Here's the drawing with two shaded views (mm, measured from the low corner). I have some questions. Coordinates: 2 decimals unless noted, no trailing zeros. Write each loop counter-clockwise with the first axis right and the second up, starting at its lowest first coordinate (ties: lowest second). Pieces come first, ordered by that corner, then holes. Notation, with made-up numbers: (72.25, -25.5) - (126.25, -25.5) arc R7 ccw to (126.25, -13.5) - close; hole circle Ø9 at (-4, 58). An arc over 180 degrees is marked (long way). Answer in a Markdown table with one row per item. Add a question column.
Item 1: If I drill on probe 1 along X at (y, z) = (1.9, 65); probe 2 along X at (y, z) = (2.1, 63); probe 3 along X at (y, z) = (1.65, 110), over which ranges is the centre line in solid material (lowest first)? Write a range as from..to.
Item 2: Imagine slicing it at A-A (x = 45). Please give me the cut outline in (y, z).
Item 3: Imagine slicing it at D-D (z = 14). Please give me the cut outline in (x, y), plus the area to 3 significant figures.
Item 4: Imagine slicing it at B-B (y = 2). State how many separate pieces and enclosed holes the cut face has, plus the area to 3 significant figures.
Item 5: I'm going to push a flat-ended pin straight in: pin 1 (10 mm diameter, centred on x = 34, z = 31.5, fed in from -Y). Where does the tip first touch, or does it pass through?
Item 6: Imagine slicing it at C-C (z = 65). Please give me the cut outline in (x, y).
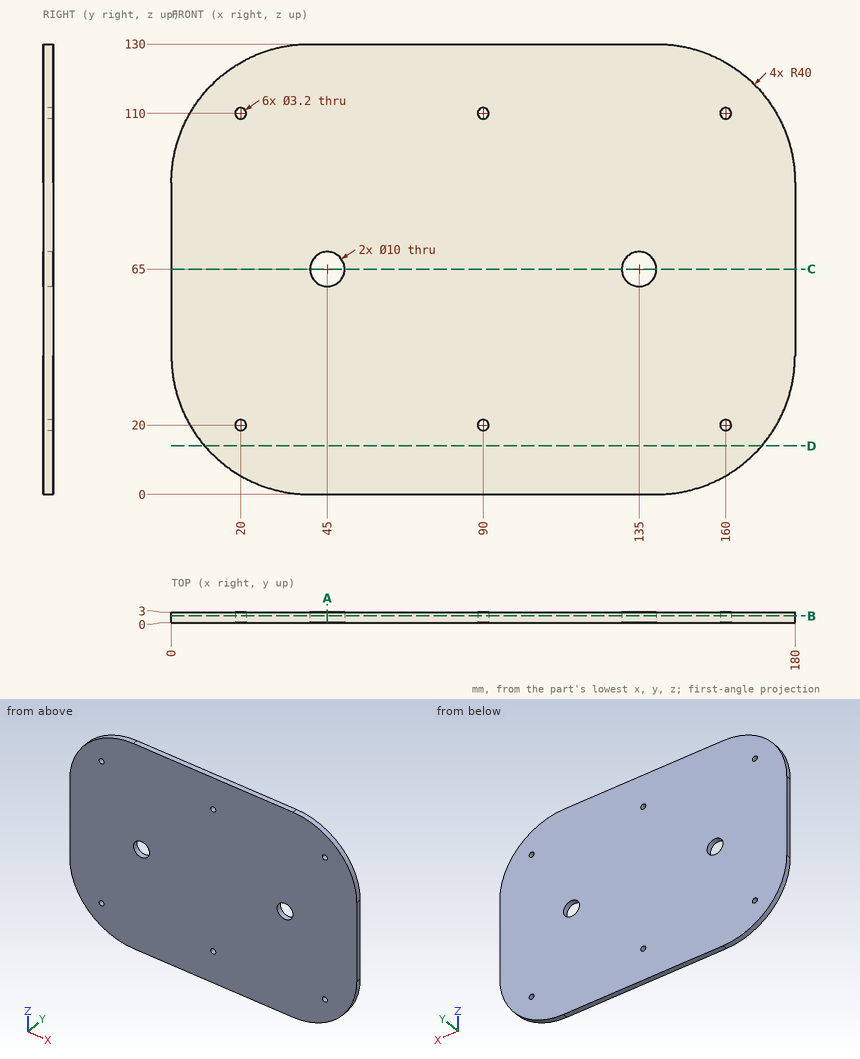
Here are the results:
| question | item | result |
|---|---|---|
| 1 | probe 1 | x = 0..40, 50..130, 140..180 |
| 1 | probe 2 | x = 0..40.42, 49.58..130.42, 139.58..180 |
| 1 | probe 3 | x = 5.36..18.4, 21.6..88.4, 91.6..158.4, 161.6..174.64 |
| 2 | outline | (0, 0) - (3, 0) - (3, 60) - (0, 60) - close; (0, 70) - (3, 70) - (3, 130) - (0, 130) - close |
| 3 | outline | (9.6, 0) - (170.4, 0) - (170.4, 3) - (9.6, 3) - close |
| 3 | area | 482 mm2 |
| 4 | separate pieces | 1 |
| 4 | enclosed holes | 8 |
| 4 | area | 21,800 mm2 |
| 5 | pin 1 | stops at y = 0 |
| 6 | outline | (0, 0) - (40, 0) - (40, 3) - (0, 3) - close; (50, 0) - (130, 0) - (130, 3) - (50, 3) - close; (140, 0) - (180, 0) - (180, 3) - (140, 3) - close |
